The listing builds one solid part. Answer for the finished solid, in the listing's coordinates (mm). A direction names the side the tool comes from. Coordinates: 2 decimals unless noted, no trailing zeros. Loops run counter-clockwise (first coordinate to the right, second up) from the corner with the lowest first, then second, coordinate; pieces in that order, holes last. Notation, with made-up numbers: (-32, -14) -> (-12, -14) arc R35 ccw to (-12, 24) -> close; hole circle Ø5 at (33.25, 6.5). An arc over 180 degrees is marked (long way). Answer in a Markdown table with one row per item.
```python
from build123d import *

# Parameters (mm, degrees)
F1_DEPTH = 63.5
F0_W     = 25.4
F0_H     = 19.05
F2_DEPTH = 25.4
F3_DEPTH = 7.9375
F5_R     = 6.35


# Not quite as in the source:
# - a feature names something its author has since deleted; it is built from what else it names


with BuildPart() as f1:
    # F0 (on Front) → F1 (new body, symmetric)
    with BuildSketch(Plane.XZ):
        Polygon((41.275, -9.525), (41.275, 9.525), (22.225, 9.525), (-41.275, 9.525), (-41.275, -9.525), align=None)
    extrude(amount=F1_DEPTH, both=True)

    # F0 (on Front) → F2 (join, symmetric)
    with BuildSketch(Plane.XZ):
        with BuildLine():
            Line((22.225, 9.525), (41.275, 9.525))
            Line((41.275, 9.525), (41.275, 27.0002))
            ThreePointArc((41.275, 27.0002), (45.9246798487, 38.2255201513), (57.15, 42.8752))
            Line((57.15, 42.8752), (60.325, 42.8752))
            Line((60.325, 42.8752), (60.325, 61.9252))
            Line((60.325, 61.9252), (57.15, 61.9252))
            ThreePointArc((57.15, 61.9252), (32.4542956671, 51.6959043329), (22.225, 27.0002))
            Line((22.225, 27.0002), (22.225, 9.525))
        make_face()
        with Locations((73.025, 52.4002)):
            Rectangle(F0_W, F0_H)
    extrude(amount=F2_DEPTH, both=True)

    # F0 (on Front) → F3 (join, symmetric)
    with BuildSketch(Plane.XZ):
        with BuildLine():
            Line((-41.275, 9.525), (22.225, 9.525))
            Line((22.225, 9.525), (22.225, 27.0002))
            ThreePointArc((22.225, 27.0002), (32.4542956671, 51.6959043329), (57.15, 61.9252))
            add(Edge.make_bspline(
                [(-41.275, 9.525), (7.2152586654, 16.9252250344), (10.756178759, 66.7510330677), (57.15, 61.9252)],
                knots=[0, 0, 0, 0, 111.5045361635, 111.5045361635, 111.5045361635, 111.5045361635], degree=3))
        make_face()
    extrude(amount=F3_DEPTH, both=True)

    # F0 (on Front) → F4 (revolve)
    with BuildSketch(Plane.XZ):
        Polygon((85.725, 61.9252), (85.725, 42.8752), (85.725, 38.1), (111.125, 38.1), (111.125, 66.675), (85.725, 66.675), align=None)
    revolve(axis=Axis((85.725, 0, 52.3875), (0, 0, -1)))

    # F5
    f5_edges = [f1.edges().sort_by_distance(p)[0] for p in [
        (41.275, -63.5, 0),
        (-41.275, -63.5, 0),
        (41.275, 63.5, 0),
        (-41.275, 63.5, 0),
    ]]
    fillet(f5_edges, radius=F5_R)


solid = f1.part
```
Item 1: A cutting plane is placed at A-A, the plane z = 1.5. Determine the outline of the cut face in (x, y) (3 decimals), plus the area to 3 significant figures.
Findings below:
| item | result |
|---|---|
| outline | (-41.275, -57.15) arc R6.35 ccw to (-34.925, -63.5) -> (34.925, -63.5) arc R6.35 ccw to (41.275, -57.15) -> (41.275, 57.15) arc R6.35 ccw to (34.925, 63.5) -> (-34.925, 63.5) arc R6.35 ccw to (-41.275, 57.15) -> close |
| area | 10,400 mm2 |
Item 2: A cutting plane is placed at B-B, the plane y = -44.5. Determine the outline of the cut face in (x, z) (3 decimals).
Findings below:
| item | result |
|---|---|
| outline | (-41.275, -9.525) -> (41.275, -9.525) -> (41.275, 9.525) -> (-41.275, 9.525) -> close |
Item 3: Find the intervals of material crossed by probe 1 along X at (y, z) = (3.5, 6) (3 decimals); probe 2 along Z at (x, y) = (-29.5, 17.5) (3 decimals); probe 3 along Z at (x, y) = (93, -4.5) (3 decimals), in increasing order.
Findings below:
| item | result |
|---|---|
| probe 1 | x = -41.275 to 41.275 |
| probe 2 | z = -9.525 to 9.525 |
| probe 3 | z = 38.1 to 66.675 |
Item 4: A cutting plane is placed at C-C, the plane x = 96.5. Determine the outline of the cut face in (y, z) (3 decimals), plus the area to 3 significant figures.
Findings below:
| item | result |
|---|---|
| outline | (-23.001, 38.1) -> (23.001, 38.1) -> (23.001, 66.675) -> (-23.001, 66.675) -> close |
| area | 1,310 mm2 |
Item 5: A tool of negligible diameter and unlimited length cuts with its end or side. For faces 1 (the face through (8, -7.938, 26)), 2 (the face through (60, 2, 42.875)), 3 (the face through (60, -2, 61.925)), 4 (the face through (41.275, -1, 4)), 5 (the face through (0, -63.5, 0)), from which of +Z, -Z, +X, -X, +Y, -Y can it reach the whole face along a straight path? Write none if from no direction.
Findings below:
| item | result |
|---|---|
| face 1 | +Z, -X, -Y |
| face 2 | -Z |
| face 3 | +Z |
| face 4 | -Z, +X, +Y, -Y |
| face 5 | +Z, -Z, +X, -X, -Y |
Item 6: Flat-ended cylindrical pins translate along their axes: pin 1 Ø5 at (y, z) = (-8.5, 28) entering from +X; pin 2 Ø16 at (x, z) = (-12, 36) entering from -Y; pin 3 Ø5 at (y, z) = (10, -1) entering from +X (3 decimals); pin 4 Ø8 at (y, z) = (25.5, 45.5) entering from +X. Find the tip coordinate at first contact, or state that the pin passes through.
Findings below:
| item | result |
|---|---|
| pin 1 | stops at x = 41.67 |
| pin 2 | passes through |
| pin 3 | stops at x = 41.275 |
| pin 4 | stops at x = 99.25 |
Item 7: Determine the mould class of faces 6 (the face through (86, 0, 38.1)), 7 (the face through (22.225, -17, 18)), 8 (the face through (39.464, -61.59, 0.133)), 9 (the face through (45.8, -0.4, 38.1)) for opening direction X: +X half, -X half, draft (parallel to the pull), parting line (faces both ways), or undercut.
Findings below:
| item | result |
|---|---|
| face 6 | draft |
| face 7 | -X half |
| face 8 | +X half |
| face 9 | undercut |
